Autodesk Inventor part; units mm, degrees
ref_plane "YZ Plane" through (0, 0, 0) normal (1, 0, 0) x (0, 1, 0)
ref_plane "XZ Plane" through (0, 0, 0) normal (0, 1, 0) x (-1, 0, 0)
ref_plane "XY Plane" through (0, 0, 0) normal (0, 0, 1) x (1, 0, 0)
sketch "Sketch1" plane through (0, 0, 0) normal (0, 1, 0) x (-1, 0, 0)
  line L0 (0, 0) -> (60, 0)
  line L1 (60, 0) -> (60, -24)
  line L2 (60, -24) -> (40, -24)
  line L3 (40, -24) -> (40, -100)
  line L4 (40, -100) -> (60, -100)
  line L5 (60, -100) -> (60, -124)
  line L6 (60, -124) -> (0, -124)
  line L7 (0, -124) -> (0, 0)
  dimension "d0" = 60
  dimension "d1" = 24
  dimension "d2" = 20
  dimension "d3" = 76
  dimension "d4" = 20
  dimension "d5" = 24
extrude "Extrusion1" add sketch "Sketch1" along normal blind 1
sketch "Sketch2" plane through (0, 1, 0) normal (0, 1, 0) x (1, 0, 0)
  circle A0 centre (-52, 6) radius 2.2
  line L0 (-60, 0) -> (0, 0)
  line L1 (-60, 24) -> (-60, 0)
  circle A1 centre (-52, 18) radius 2.2
  line L2 (-48.25, 3) -> (-37.25, 3)
  line L3 (-37.25, 3) -> (-37.25, 21)
  line L4 (-37.25, 21) -> (-48.25, 21)
  line L5 (-48.25, 21) -> (-48.25, 3)
  circle A2 centre (-34, 17.9998) radius 2.2
  circle A3 centre (-33.9323, 6) radius 2.2
  line L6 (-40, 100) -> (-40, 24)
  line L7 (-40, 62) -> (0, 62)
  circle A4 centre (-52, 118) radius 2.2
  circle A5 centre (-52, 106) radius 2.2
  line L8 (-48.25, 121) -> (-37.25, 121)
  line L9 (-37.25, 121) -> (-37.25, 103)
  line L10 (-37.25, 103) -> (-48.25, 103)
  line L11 (-48.25, 103) -> (-48.25, 121)
  circle A6 centre (-34, 106.0002) radius 2.2
  circle A7 centre (-33.9323, 118) radius 2.2
  line L12 (-60, 124) -> (0, 124)
  line L13 (-60, 124) -> (-60, 100)
  dimension "d8" = 4.4
  dimension "d9" = 6
  dimension "d10" = 8
  dimension "d11" = 4.4
  dimension "d12" = 12
  dimension "d13" = 11
  dimension "d14" = 18
  dimension "d15" = 3
  dimension "d16" = 3.75
  dimension "d17" = 4.4
  dimension "d18" = 3.25
  dimension "d19" = 4.4
  dimension "d20" = 6
  dimension "d21" = 8
  dimension "d22" = 8
extrude "Extrusion2" cut sketch "Sketch2" against normal blind 1.5
sketch "Sketch4" plane through (0, 1, 0) normal (0, 1, 0) x (1, 0, 0)
  line L0 (-60, 124) -> (-60, 100)
  line L1 (-60, 100) -> (-60, 97.5)
  line L2 (-60, 97.5) -> (-40, 97.5)
  line L3 (-40, 100) -> (-40, 24)
  line L4 (-40, 24) -> (-60, 24)
  line L5 (-60, 24) -> (-60, 26.5)
  line L6 (-60, 26.5) -> (-40, 26.5)
  line L7 (-40, 100) -> (-60, 100)
  line L8 (-40, 24) -> (-40, 100)
  line L9 (-60, 100) -> (-40, 100)
  line L10 (-40, 100) -> (-40, 97.5)
  line L11 (-60, 24) -> (-40, 24)
  line L12 (-40, 26.5) -> (-40, 24)
  line L13 (-60, 124) -> (-41.5, 124)
  line L14 (0, 124) -> (-60, 124)
  line L15 (-41.5, 124) -> (-41.5, 126)
  line L16 (-41.5, 126) -> (-24, 126)
  line L17 (-24, 126) -> (-24, 124)
  line L18 (-41.5, 124) -> (-24, 124)
  line L19 (-40, 62) -> (-22.3006, 62)
  line L20 (0, 0) -> (-60, 0)
  line L21 (-41.5, 0) -> (-41.5, -2)
  line L22 (-41.5, -2) -> (-24, -2)
  line L23 (-24, -2) -> (-24, 0)
  line L24 (-60, 0) -> (0, 0)
  dimension "d29" = 2.5
  dimension "d30" = 2.5
  dimension "d32" = 18.5
  dimension "d33" = 2
  dimension "d34" = 17.5
extrude "Extrusion3" add sketch "Sketch4" along normal blind 24 and the other way blind 1
sketch "Sketch6" plane through (-24, 25, -126) normal (0, 0, -1) x (-1, 0, 0)
  circle A0 centre (4, -6) radius 2.2
  line L0 (0, -25) -> (0, 0)
  line L1 (0, 0) -> (17.5, 0)
  circle A1 centre (4, -12) radius 2.2
  circle A2 centre (4, -18) radius 2.2
  line L2 (0, 0) -> (0, -24)
  line L3 (17.5003, -24) -> (0, -24)
  point P0 (-24, -25)
  dimension "d39" = 4.4
  dimension "d40" = 4
  dimension "d41" = 6
  dimension "d42" = 4.4
  dimension "d43" = 4.4
  dimension "d44" = 6
  dimension "d45" = 6
  dimension "d46" = 6
hole "Hole1" at (-28, 7, -126) at (-28, 13, -126) at (-28, 19, -126) direction (0, 0, 1) diameter 4.4 depth 2
sketch "Sketch7" plane through (-41.5, 25, 2) normal (0, 0, 1) x (1, 0, 0)
  line L0 (17.5, -24) -> (0, -24)
  line L1 (0, -24) -> (0, -25)
  line L2 (17.5, -24) -> (0, -24)
  circle A0 centre (13.5, -18) radius 2.2
  circle A1 centre (13.5, -18) radius 2.2
  circle A2 centre (13.5, -12) radius 2.2
  circle A3 centre (13.5, -12) radius 2.2
  circle A4 centre (13.5, -6) radius 2.2
  circle A5 centre (13.5, -6) radius 2.2
  point P0 (41.5, -25)
  dimension "d54" = 4.4
  dimension "d55" = 4.4
  dimension "d56" = 4.4
hole "Hole2" at (-28, 7, 2) at (-28, 13, 2) at (-28, 19, 2) direction (0, 0, -1) diameter 4.4 depth 2
sketch "Sketch11" plane through (-60, 1, -100) normal (0, 0, -1) x (-1, 0, 0)
  circle A0 centre (-8, 18) radius 2.2
  line L0 (0, 24) -> (0, 0)
  line L1 (-20, 24) -> (0, 24)
  circle A1 centre (-8, 12) radius 2.2
  circle A2 centre (-8, 6) radius 2.2
  circle A3 centre (-31.5, 6) radius 2.2
  circle A4 centre (-31.5, 12) radius 2.2
  circle A5 centre (-31.5, 18) radius 2.2
  point P0 (-60, -1)
  point P1 (-36, 24)
  dimension "d68" = 4.4
  dimension "d69" = 8
  dimension "d70" = 6
  dimension "d71" = 4.4
  dimension "d72" = 4.4
  dimension "d73" = 6
  dimension "d74" = 6
  dimension "d82" = 4.4
  dimension "d83" = 23.5
  dimension "d84" = 4.4
  dimension "d85" = 4.4
hole "Hole3" at (-52, 19, -100) at (-52, 13, -100) at (-52, 7, -100) direction (0, 0, 1) diameter 4.4 depth 2.5
sketch "Sketch12" plane through (-60, 1, -24) normal (0, 0, 1) x (1, 0, 0)
  circle A0 centre (8, 6) radius 2.2
  circle A1 centre (8, 6) radius 2.2
  circle A2 centre (8, 12) radius 2.2
  circle A3 centre (8, 12) radius 2.2
  circle A4 centre (8, 18) radius 2.2
  circle A5 centre (8, 18) radius 2.2
  point P0 (60, -1)
  dimension "d86" = 4.4
  dimension "d87" = 4.4
  dimension "d88" = 4.4
hole "Hole4" at (-52, 7, -24) at (-52, 13, -24) at (-52, 19, -24) direction (0, 0, -1) diameter 4.4 depth 2.5
sketch "Sketch13" plane through (-60, 1, -24) normal (0, 0, 1) x (1, 0, 0)
  point P0 (60, -1)
properties part number "brace"
Source: CAD feature listing. Evaluate the final solid. Frame: model axes, mm. A direction names the side the tool comes from. Round coordinates to 2 decimals unless told otherwise and drop trailing zeros. Loops run counter-clockwise (first coordinate to the right, second up) from the corner with the lowest first, then second, coordinate; pieces in that order, holes last.
1. Ray query, L1, parallel to Y at x = -28, z = -125.3; L2, parallel to X at y = 0.4, z = -6; L3, parallel to Z at x = -52, y = 0.6. Return the intervals inside material, ascending.
2. Access query for faces 1 (the flat face through (-33, 13, 0)), 2 (the cylindrical face through (-54.198, 0.507, -18.097)), 3 (the flat face through (-40, 13, -99)). Directions: +Z, -Z, +X, -X, +Y, -Y. A direction counts if a zero-diameter tool reaches every point of the face in a straight line with its end or side. Return the directions, or none.
3. Section query A-A on z = -6. Output: boundary loops of the cut face in (x, y).
4. Mould query, pull axis Y, two halves, no side actions, for faces 4 (the flat face through (-48, 12, -97.5)), 5 (the cylindrical face through (-49.852, 12.523, -98.732)), 6 (the flat face through (-50, 25, -99)), 7 (the cylindrical face through (-49.852, 6.523, -98.732)). Classes: released by +Y, released by -Y, zero draft, split by the parting line, or undercut.
5. Contact query for flat-ended pins moving along their axis: pin 1 (3.5 mm diameter, centred on x = -52, y = 7, fed in from +Z); pin 2 (0.8 mm diameter, centred on x = -50, y = 0.5, fed in from -Z); pin 3 (3 mm diameter, centred on y = 11.5, z = -99, fed in from +X); pin 4 (1 mm diameter, centred on y = 7, z = -125, fed in from -X). Output: stop coordinate, or through.
6. Section query B-B on y = 13. Give the number of separate pieces and of enclosed holes in the cut face, and give its area (3 significant figures).
7. Section query D-D on x = -34. Output: boundary loops of the cut face in (y, z), and give its area (3 significant figures).
Answers below:
1. L1: y = 0 to 4.8, 9.2 to 10.8, 15.2 to 16.8, 21.2 to 25
1. L2: x = -60 to -54.2, -49.8 to -48.25, -37.25 to -36.13, -31.73 to 0
1. L3: z = -124 to -120.2, -115.8 to -108.2, -103.8 to -97.5, -26.5 to -20.2, -15.8 to -8.2, -3.8 to 0
2. face 1: +X, -X, +Y
2. face 2: +Y, -Y
2. face 3: +X, +Y
3. outline: (-60, 0) - (-54.2, 0) - (-54.2, 1) - (-60, 1) - close; (-49.8, 0) - (-48.25, 0) - (-48.25, 1) - (-49.8, 1) - close; (-37.25, 0) - (-36.13, 0) - (-36.13, 1) - (-37.25, 1) - close; (-31.73, 0) - (0, 0) - (0, 1) - (-31.73, 1) - close
4. face 4: zero draft
4. face 5: undercut
4. face 6: released by +Y
4. face 7: undercut
5. pin 1: passes through
5. pin 2: stops at z = -124
5. pin 3: stops at x = -40
5. pin 4: stops at x = -41.5
6. separate pieces: 8
6. enclosed holes: 0
6. area: 130 mm2
7. outline: (0, -126) - (25, -126) - (25, -124) - (1, -124) - (1, -120.2) - (0, -120.2) - close; (0, -115.8) - (1, -115.8) - (1, -108.2) - (0, -108.2) - close; (0, -103.8) - (1, -103.8) - (1, -20.2) - (0, -20.2) - close; (0, -15.8) - (1, -15.8) - (1, -8.2) - (0, -8.2) - close; (0, -3.8) - (1, -3.8) - (1, 0) - (25, 0) - (25, 2) - (0, 2) - close
7. area: 206 mm2
